For this review, take the finished solid that the model builds, in its own axes (mm). A direction names the side the tool comes from. Give positions to 0.01 mm unless a question says otherwise; leave off trailing zeros. Write each loop counter-clockwise with the first axis right and the second up, starting at its lowest first coordinate (ties: lowest second). Pieces come first, ordered by that corner, then holes.
Q1. For line 1 (Y direction, x = -7.5, z = 0.35); line 2 (X direction, y = 7, z = 0.75); line 3 (X direction, y = -37.5, z = 0.8), list the stretches that pass through material, from the lowest coordinate up.
Q2. We need section D-D (x = -41). Write out the cut boundary in (y, z).
Q3. We need section A-A (z = 0.8). Write out the cut boundary in (x, y), then the cut area to 3 significant figures.
Q4. Mouldability with a two-part tool opening along Y and no side actions: class faces 6 (the flat face through (21, 0, 1)), 7 (the cylindrical face through (-43.22, 40.74, 1.48)), 8 (the flat face through (47.5, -17, 1)) as released by +Y, released by -Y, zero draft, split by the parting line, or undercut.
Q5. We need section B-B (x = -0.5). Write out the cut boundary in (y, z).
Q6. Machinability: for faces 1 (the flat face through (-2, -42.25, 1)), 2 (the flat face through (-21, 0, 1)), 3 (the flat face through (-44.5, -1, 1)), 4 (the flat face through (-2, 42.25, 1)), 5 (the flat face through (46, -4.25, 1)), which of the approach directions +Z, -Z, +X, -X, +Y, -Y give a long, thin tool a straight path to every point of the face, cutting with its end or side? Answer none if there is none.
Q7. Insertion check: P1, Ø1.5, axis at y = -2, z = 1.5, coming from the -X side; P2, Ø0.9, axis at x = -1, z = 1, coming from the +Y side; P3, Ø0.9, axis at y = 44.5, z = 1.5, coming from the +X side. Each pin has a flat end and moves straight along its axis. Give the tip position at first contact, or say it passes through.
Q8. We need section C-C (x = 40.5). Write out the cut boundary in (y, z), then the cut area to 3 significant figures.
```python
from build123d import *

# Parameters (mm, degrees)
SKETCH1_W           = 42
SKETCH1_H           = 40.010526316
BOSS_EXTRUDE1_DEPTH = 3


with BuildPart() as part:
    # Sketch1 → Boss-Extrude1 (new body)
    with BuildSketch(Plane.XY):
        with BuildLine():
            Line((-47.5, -4.25), (-44.5, -4.25))
            Line((-44.5, -4.25), (-44.5, 1.95))
            Line((-44.5, 1.95), (-47.5, 1.95))
            Line((-47.5, 1.95), (-47.5, 30.25))
            ThreePointArc((-47.5, 30.25), (-43.106601718, 40.856601718), (-32.5, 45.25))
            Line((-32.5, 45.25), (-4.75, 45.25))
            Line((-4.75, 45.25), (-4.75, 42.25))
            Line((-4.75, 42.25), (1.25, 42.25))
            Line((1.25, 42.25), (1.25, 45.25))
            Line((1.25, 45.25), (32.5, 45.25))
            ThreePointArc((32.5, 45.25), (43.106601718, 40.856601718), (47.5, 30.25))
            Line((47.5, 30.25), (47.5, 1.95))
            Line((47.5, 1.95), (44.5, 1.95))
            Line((44.5, 1.95), (44.5, -4.25))
            Line((44.5, -4.25), (47.5, -4.25))
            Line((47.5, -4.25), (47.5, -30.25))
            ThreePointArc((47.5, -30.25), (43.106601718, -40.856601718), (32.5, -45.25))
            Line((32.5, -45.25), (1.25, -45.25))
            Line((1.25, -45.25), (1.25, -42.25))
            Line((1.25, -42.25), (-4.75, -42.25))
            Line((-4.75, -42.25), (-4.75, -45.25))
            Line((-4.75, -45.25), (-32.5, -45.25))
            ThreePointArc((-32.5, -45.25), (-43.106601718, -40.856601718), (-47.5, -30.25))
            Line((-47.5, -30.25), (-47.5, -4.25))
        make_face()
        Rectangle(SKETCH1_W, SKETCH1_H, mode=Mode.SUBTRACT)
    extrude(amount=BOSS_EXTRUDE1_DEPTH)


solid = part.part
```
Computed:
1. line 1: y = -45.25 to -20.01, 20.01 to 45.25
1. line 2: x = -47.5 to -21, 21 to 47.5
1. line 3: x = -45.63 to 45.63
2. outline: (-42.61, 0) - (42.61, 0) - (42.61, 3) - (-42.61, 3) - close
3. outline: (-47.5, -30.25) arc R15 ccw to (-32.5, -45.25) - (-4.75, -45.25) - (-4.75, -42.25) - (1.25, -42.25) - (1.25, -45.25) - (32.5, -45.25) arc R15 ccw to (47.5, -30.25) - (47.5, -4.25) - (44.5, -4.25) - (44.5, 1.95) - (47.5, 1.95) - (47.5, 30.25) arc R15 ccw to (32.5, 45.25) - (1.25, 45.25) - (1.25, 42.25) - (-4.75, 42.25) - (-4.75, 45.25) - (-32.5, 45.25) arc R15 ccw to (-47.5, 30.25) - (-47.5, 1.95) - (-44.5, 1.95) - (-44.5, -4.25) - (-47.5, -4.25) - close; hole (-21, -20.01) - (21, -20.01) - (21, 20.01) - (-21, 20.01) - close
3. area: 6,650 mm2
4. face 6: undercut
4. face 7: released by +Y
4. face 8: zero draft
5. outline: (-42.25, 0) - (-20.01, 0) - (-20.01, 3) - (-42.25, 3) - close; (20.01, 0) - (42.25, 0) - (42.25, 3) - (20.01, 3) - close
6. face 1: +Z, -Z, -Y
6. face 2: +Z, -Z
6. face 3: +Z, -Z, -X
6. face 4: +Z, -Z, +Y
6. face 5: +Z, -Z, +X
7. P1: stops at x = -44.5
7. P2: stops at y = 42.25
7. P3: stops at x = 38.38
8. outline: (-42.94, 0) - (42.94, 0) - (42.94, 3) - (-42.94, 3) - close
8. area: 258 mm2
